```python
from build123d import *

# Parameters (mm, degrees)
SKETCH2_R = 25
SHELL1_T  = -3


with BuildPart() as part:
    # Sweep1: sweep along a path in Sketch1
    with BuildLine(Plane.XY) as sweep1_path:
        Line((0, 0), (0, 100))
        ThreePointArc((0, 100), (23.431457505, 156.568542495), (80, 180))
    # Sketch2 → Sweep1 (sweep)
    with BuildSketch(Plane(origin=(0, 0, 0), x_dir=(1, 0, 0), z_dir=(0, 1, 0))):
        Circle(SKETCH2_R)
    sweep(path=sweep1_path.line)

    # Shell1
    shell1_openings = [part.faces().sort_by_distance(p)[0] for p in [
        (0, 0, 0),
    ]]
    offset(amount=SHELL1_T, openings=shell1_openings, kind=Kind.INTERSECTION)


solid = part.part
```
For this review, take the finished solid that the model builds, in its own axes (mm). Round coordinates to 2 decimals unless told otherwise and drop trailing zeros. Loops run counter-clockwise (first coordinate to the right, second up) from the corner with the lowest first, then second, coordinate; pieces in that order, holes last.
Q1. Add section B-B on y = 89. Write out the cut boundary in (x, z).
Result sheet:
outline: circle Ø50 at (0, 0); hole circle Ø44 at (0, 0)
Q2. Add section A-A on z = 0. Write out the cut boundary in (x, y).
Result sheet:
outline: (-25, 0) - (-22, 0) - (-22, 100) arc R102 cw to (77, 201.96) - (77, 157.92) arc R58 ccw to (22, 100) - (22, 0) - (25, 0) - (25, 100) arc R55 cw to (80, 155) - (80, 205) arc R105 ccw to (-25, 100) - close
Q3. Insertion check: pin 1 Ø1.5 at (x, z) = (44.5, -5.5) entering from +Y; pin 2 Ø1.5 at (y, z) = (60, -14.5) entering from +X; pin 3 Ø8 at (x, z) = (58, -6) entering from -Y. Each pin has a flat end and moves straight along its axis. Give the tip position at first contact, or say it passes through.
Result sheet:
pin 1: stops at y = 198.48
pin 2: stops at x = 20.88
pin 3: stops at y = 149.08
Q4. To check wall thickness, follow line 1 along Z through (x, y) = (0, 54); line 2 along Y through (x, z) = (57, -18). State the ranges of each line that lie inside material, in increasing order.
Result sheet:
line 1: z = -25 to -22, 22 to 25
line 2: y = 158.28 to 163.3, 189.75 to 194.59
Q5. Add section C-C on z = 15. Write out the cut boundary in (x, y), plus the area to 3 significant figures.
Result sheet:
outline: (-20, 0) - (-16.09, 0) - (-16.09, 100) arc R96.09 cw to (77, 196.05) - (77, 163.84) arc R63.91 ccw to (16.09, 100) - (16.09, 0) - (20, 0) - (20, 100) arc R60 cw to (80, 160) - (80, 200) arc R100 ccw to (-20, 100) - close
area: 1,860 mm2
Q6. Mouldability with a two-part tool opening along Y and no side actions: class faces 1 (the face through (-22.1, 0, 1.7)), 2 (the face through (80, 180, 0)), 3 (the face through (77, 180, 0)) as +Y half, -Y half, draft (parallel to the pull), parting line (faces both ways), or undercut.
Result sheet:
face 1: -Y half
face 2: draft
face 3: undercut
